The listing builds one solid part. Answer for the finished solid, in the listing's coordinates (mm). Round coordinates to 2 decimals unless told otherwise and drop trailing zeros. Write each loop counter-clockwise with the first axis right and the second up, starting at its lowest first coordinate (ties: lowest second). Pieces come first, ordered by that corner, then holes.
(1) A cutting plane is placed at D-D, the plane y = -18. Give the vertices of the cut face in (x, z), and give its area (3 significant figures).
(2) Find the intervals of material crossed by probe 1 along Y at (x, z) = (-14.5, 1.8); probe 2 along Y at (x, z) = (-27, 0.4) (3 decimals); probe 3 along X at (y, z) = (9.5, 0.15), in increasing order.
(3) A cutting plane is placed at A-A, the plane y = -27.5. Give the vertices of the cut face in (x, z).
(4) A cutting plane is placed at B-B, the plane x = -20. Give the vertices of the cut face in (y, z).
(5) Each of these flat-tipped pins is pushed along its axis until it touches: pin 1 Ø3 at (x, y) = (0, -12.02) entering from +Z; pin 2 Ø1.5 at (y, z) = (-26, 1.5) entering from -X; pin 3 Ø3 at (x, y) = (19.5, -24.5) entering from -Z; pin 4 Ø1 at (x, z) = (-25.5, 2) entering from +Y. Where does it stop, or does it pass through?
(6) A cutting plane is placed at C-C, the plane y = 0. Give the vertices of the cut face in (x, z).
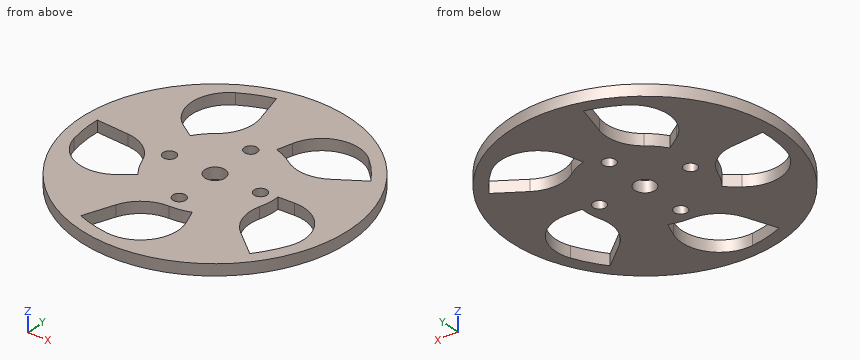
Autodesk Inventor part; units mm, degrees
ref_plane "YZ Plane" through (0, 0, 0) normal (1, 0, 0) x (0, 1, 0)
ref_plane "XZ Plane" through (0, 0, 0) normal (0, 1, 0) x (-1, 0, 0)
ref_plane "XY Plane" through (0, 0, 0) normal (0, 0, 1) x (1, 0, 0)
sketch "Sketch1" plane through (0, 0, 0) normal (0, 0, 1) x (1, 0, 0)
  circle A0 centre (0, 0) radius 35.75
  circle A1 centre (0, 0) radius 32.5
  circle A2 centre (0, 0) radius 16
  circle A3 centre (0, 0) radius 2.7
  line L0 (0, 0) -> (-8.4116, 31.3926)
  line L1 (0, 0) -> (8.4116, 31.3926)
  line L2 (0, 0) -> (0, 4.5704)
  line L3 (0, 0) -> (-32.4555, 1.7009)
  line L4 (0, 0) -> (-27.2568, 17.7008)
  line L5 (0, 0) -> (-11.647, -30.3414)
  line L6 (0, 0) -> (-25.2572, -20.4529)
  line L7 (0, 0) -> (25.2572, -20.4529)
  line L8 (0, 0) -> (11.647, -30.3414)
  line L9 (0, 0) -> (27.2568, 17.7008)
  line L10 (0, 0) -> (32.4555, 1.7009)
  point P0 (4.1411, 15.4548)
  point P1 (13.4187, 8.7142)
  point P2 (-4.1411, 15.4548)
  point P3 (-13.4187, 8.7142)
  point P4 (12.4343, -10.0691)
  point P5 (15.9781, 0.8374)
  point P6 (-5.7339, -14.9373)
  point P7 (5.7339, -14.9373)
  point P8 (-15.9781, 0.8374)
  point P9 (-12.4343, -10.0691)
  dimension "d0" = 71.5
  dimension "d1" = 65
  dimension "d2" = 5.4
  dimension "d3" = 32
  dimension "d4" = 15
  dimension "d5" = 15
  dimension "d8" = 360
extrude "Extrusion1" add sketch "Sketch1" along normal blind 3 contours A0 | L10 A2 L9 A1 | A1 L8 A2 L7 | L10 A3 L9 A2 | A2 L7 A3 L10 | A2 L8 A3 L7 | L1 A2 L0 A1 | L9 A3 L1 A2 | A1 L6 A2 L5 | A2 L5 A3 L8 | L1 A3 L0 A2 | A2 L6 A3 L5 | L4 A2 L3 A1 | L0 A3 L4 A2 | L3 A2 L4 A3 | A3 L6 A2 L3
fillet "Fillet1" radius 10 10 edges at (8.4116, 31.3926, 1.5) (-27.2568, 17.7008, 1.5) (-25.2572, -20.4529, 1.5) (11.647, -30.3414, 1.5) (32.4555, 1.7009, 1.5) (-15.9781, 0.8374, 1.5) (-4.1411, 15.4548, 1.5) (13.4187, 8.7142, 1.5) (12.4343, -10.0691, 1.5) (-5.7339, -14.9373, 1.5)
sketch "Sketch2" plane through (0, 0, 3) normal (0, 0, 1) x (1, 0, 0)
  circle A0 centre (0, 12.0208) radius 1.7
  circle A1 centre (-12.0208, 0) radius 1.7
  circle A2 centre (0, -12.0208) radius 1.7
  circle A3 centre (12.0208, 0) radius 1.7
  line L0 (0, 12.0208) -> (-12.0208, 0)
  line L1 (-12.0208, 0) -> (0, -12.0208)
  line L2 (0, -12.0208) -> (12.0208, 0)
  line L3 (12.0208, 0) -> (0, 12.0208)
  point P0 (0, 0)
  dimension "d13" = 17
  dimension "d14" = 17
  dimension "d15" = 3.4
  dimension "d16" = 3.4
  dimension "d17" = 3.4
  dimension "d18" = 3.4
extrude "Extrusion2" cut sketch "Sketch2" against normal blind 3 contours A0 L3 L0 | L0 L3 A0 | L0 L1 A1 | A1 L1 L0 | L3 L2 A3 | A3 L2 L3 | L1 L2 A2 | A2 L2 L1
properties part number "Wheel_2D_Int"
Solutions:
1. outline: (-30.89, 0) - (-5.28, 0) - (-5.28, 3) - (-30.89, 3) - close; (6.91, 0) - (22.23, 0) - (22.23, 3) - (6.91, 3) - close; (27.06, 0) - (30.89, 0) - (30.89, 3) - (27.06, 3) - close
1. area: 134 mm2
2. probe 1: y = -32.68 to -11.74, -6.76 to 9.42, 29.09 to 32.68
2. probe 2: y = -23.432 to -13.548, 1.415 to 23.432
2. probe 3: x = -34.46 to -14.63, -12.87 to 34.46
3. outline: (-22.84, 0) - (-10.56, 0) - (-10.56, 3) - (-22.84, 3) - close; (6.49, 0) - (22.84, 0) - (22.84, 3) - (6.49, 3) - close
4. outline: (-29.63, 0) - (-14.72, 0) - (-14.72, 3) - (-29.63, 3) - close; (0.2, 0) - (14.17, 0) - (14.17, 3) - (0.2, 3) - close; (24.56, 0) - (29.63, 0) - (29.63, 3) - (24.56, 3) - close
5. pin 1: passes through
5. pin 2: stops at x = -25.31
5. pin 3: stops at z = 0
5. pin 4: stops at y = 25.56
6. outline: (-35.75, 0) - (-32.5, 0) - (-32.5, 3) - (-35.75, 3) - close; (-19.61, 0) - (-13.72, 0) - (-13.72, 3) - (-19.61, 3) - close; (-10.32, 0) - (-2.7, 0) - (-2.7, 3) - (-10.32, 3) - close; (2.7, 0) - (10.32, 0) - (10.32, 3) - (2.7, 3) - close; (13.72, 0) - (16, 0) - (16, 3) - (13.72, 3) - close; (25.15, 0) - (35.75, 0) - (35.75, 3) - (25.15, 3) - close
